```python
from build123d import *

# Parameters (mm, degrees)
BOSS_EXTRUDE1_DEPTH = 90
FILLET1_R           = 1


with BuildPart() as part:
    # Sketch1 → Boss-Extrude1 (new body)
    with BuildSketch(Plane(origin=(0, 0, 0), x_dir=(1, 0, 0), z_dir=(0, 1, 0))):
        with BuildLine():
            Line((-16.839290437, -36.282754823), (-10.5, -22.688102609))
            ThreePointArc((-10.5, -22.688102609), (0, 25), (10.5, -22.688102609))
            Line((10.5, -22.688102609), (16.839290437, -36.282754823))
            ThreePointArc((16.839290437, -36.282754823), (0, 40), (-16.839290437, -36.282754823))
        make_face()
    extrude(amount=BOSS_EXTRUDE1_DEPTH)

    # Fillet1
    fillet1_edges = [part.edges().sort_by_distance(p)[0] for p in [
        (0, 90, -40),
        (0, 0, -40),
    ]]
    fillet(fillet1_edges, radius=FILLET1_R)


solid = part.part
```
CAD build for the part. Positions are in the model's coordinates, mm. A direction names the side the tool comes from. Give positions to 0.01 mm unless a question says otherwise; leave off trailing zeros. Write each loop counter-clockwise with the first axis right and the second up, starting at its lowest first coordinate (ties: lowest second). Pieces come first, ordered by that corner, then holes. Notation, with made-up numbers: (60.25, 13.5) -> (92.25, 13.5) arc R16 cw to (92.25, 26.5) -> close; hole circle Ø9 at (17.5, -40). An arc over 180 degrees is marked (long way). Write each question's results on one line, items separated by ' | '.
1. Which spindle directions (+Z, -Z, +X, -X, +Y, -Y) get a long thin tool onto all of the face, cutting with end or side? Do faces 4 (the flat face through (13.625, 44.37, 29.39)), 5 (the flat face through (17, 90, -19)). Say none if no direction does.
Geometry check:
face 4: +Z, +Y, -Y | face 5: +Z, -Z, +X, -X, +Y
2. Drop flat-ended pins along their axis: P1, Ø4, axis at y = 35.5, z = 10, coming from the -X side; P2, Ø4, axis at x = 21.5, y = 48.5, coming from the +Z side; P3, Ø8, axis at y = 12.5, z = -13.5, coming from the -X side. Give the stop position or say it passes through.
Geometry check:
P1: x = -39.19 | P2: z = 34.92 | P3: x = -38.86
3. Wall check: probe 1 along X at (y, z) = (41, 0); probe 2 along Z at (x, y) = (0, 64); probe 3 along X at (y, z) = (59, -15). Give the ranges that are in metal, low to high. Write a range as [from, to].
Geometry check:
probe 1: [-40, -25], [25, 40] | probe 2: [-40, -25] | probe 3: [-37.08, -20], [20, 37.08]
4. Two-plate mould, pull along X, no slides. Class faces 1 (the cylindrical face through (1.52, 44.38, -39.97)), 2 (the flat face through (17, 0, -19)), 3 (the flat face through (-13.714, 44.37, 29.581)): pulls with the +X half, pulls with the -X half, needs draft (parallel to the pull), parting line crosses it, or undercut.
Geometry check:
face 1: parting line crosses it | face 2: needs draft | face 3: undercut
5. Cut at A-A, the plane y = 14. Write the cut outline in (x, z), then the cut area to 3 significant figures.
Geometry check:
outline: (-16.84, 36.28) arc R40 ccw (long way) to (16.84, 36.28) -> (10.5, 22.69) arc R25 cw (long way) to (-10.5, 22.69) -> close | area: 2,640 mm²
